Autodesk Inventor part; units mm, degrees
ref_plane "YZ Plane" through (0, 0, 0) normal (1, 0, 0) x (0, 1, 0)
ref_plane "XZ Plane" through (0, 0, 0) normal (0, 1, 0) x (-1, 0, 0)
ref_plane "XY Plane" through (0, 0, 0) normal (0, 0, 1) x (1, 0, 0)
sketch "Sketch1" plane through (0, 0, 0) normal (0, 1, 0) x (-1, 0, 0)
  line L0 (0, 0) -> (-50.8, 0)
  line L1 (-50.8, 0) -> (-50.8, -88.9)
  line L2 (-50.8, -88.9) -> (0, -88.9)
  line L3 (0, -88.9) -> (0, 0)
  dimension "d0" = 50.8
  dimension "d1" = 88.9
extrude "Extrusion1" add sketch "Sketch1" along normal blind 12.7
sketch "Sketch2" plane through (0, 12.7, 0) normal (0, 1, 0) x (1, 0, 0)
  line L0 (50.8, 0) -> (50.8, 88.9)
  line L1 (50.8, 88.9) -> (0, 88.9)
  line L2 (0, 88.9) -> (0, 0)
  line L3 (6.35, 88.9) -> (44.45, 88.9)
  line L4 (44.45, 88.9) -> (44.45, 69.85)
  line L5 (44.45, 69.85) -> (6.35, 69.85)
  line L6 (6.35, 69.85) -> (6.35, 88.9)
  line L7 (6.35, 79.375) -> (0, 79.375) construction
  line L8 (44.45, 79.375) -> (50.8, 79.375) construction
  circle A0 centre (25.4, 69.85) radius 19.05
  dimension "d4" = 19.05
  dimension "d5" = 6.35
extrude "Extrusion2" add sketch "Sketch2" along normal blind 12.7
sketch "Sketch3" plane through (0, 25.4, 0) normal (0, 1, 0) x (1, 0, 0)
  arc A0 (6.35, 69.85) -> (44.45, 69.85) centre (25.4, 69.85) ccw
  circle A1 centre (25.4, 69.85) radius 12.7
  point P0 (0, 0)
  dimension "d8" = 25.4
extrude "Extrusion3" add sketch "Sketch3" along normal blind 12.7
sketch "Sketch6" plane through (0, 12.7, 0) normal (0, 1, 0) x (1, 0, 0)
  line L0 (0, 88.9) -> (0, 0)
  line L1 (0, 0) -> (50.8, 0)
  line L2 (50.8, 0) -> (50.8, 88.9)
  line L3 (44.45, 88.9) -> (44.45, 6.35) construction
  line L4 (44.45, 6.35) -> (6.35, 6.35) construction
  line L5 (6.35, 6.35) -> (6.35, 88.9) construction
  line L6 (6.35, 38.1) -> (44.45, 38.1) construction
  dimension "d35" = 6.35
  dimension "d36" = 31.75
hole "Hole3" at (25.4, 38.1, -69.85) direction (0, -1, 0) diameter 19.05 end through all
hole "Hole4" at (6.35, 12.7, -6.35) at (6.35, 12.7, -38.1) at (44.45, 12.7, -6.35) at (44.45, 12.7, -38.1) direction (0, -1, 0) diameter 5.1054 end through all counterbore diameter 9.525 counterbore depth 4.826
properties part number "Holes"
Verification items for the finished model (mm, model axes). A direction names the side the tool comes from. Coordinates: 2 decimals unless noted, no trailing zeros. Loops run counter-clockwise (first coordinate to the right, second up) from the corner with the lowest first, then second, coordinate; pieces in that order, holes last. Notation, with made-up numbers: (84, -16) - (99, -16) arc R10 cw to (99, -8) - close; hole circle Ø2 at (-20.75, -20.5). An arc over 180 degrees is marked (long way). Return JSON: item names as keys, results as strings.
1. Go/stop test with flat-tipped pins: pin 1 (1 mm diameter, centred on x = 42, z = -69.5, fed in from +Y); pin 2 (6 mm diameter, centred on x = 39, z = -21, fed in from +Y); pin 3 (3 mm diameter, centred on x = 46.5, z = -38, fed in from +Y). Record where each tip stops, or that it passes through.
Established:
{"pin 1": "stops at y = 25.4", "pin 2": "stops at y = 12.7", "pin 3": "stops at y = 7.87"}
2. Tool access check on faces 1 (the flat face through (0, 6, -45)), 2 (the flat face through (44.45, 19, -80)), 3 (the flat face through (8, 7.874, -4)). Record the directions out of +Z, -Z, +X, -X, +Y, -Y that give a thin tool (end or side, any length) a straight path to the whole face; none if there is none.
Established:
{"face 1": "+Z, -Z, -X, +Y, -Y", "face 2": "+Z, -Z, +X, +Y", "face 3": "+Y"}
3. Section check D-D, the plane x = 32. Record the boundary of the cut face in (y, z), then the cut area to 3 significant figures.
Established:
{"outline": "(0, -88.9) - (25.4, -88.9) - (25.4, -80.7) - (38.1, -80.7) - (38.1, -76.72) - (0, -76.72) - close; (0, -62.98) - (38.1, -62.98) - (38.1, -59) - (25.4, -59) - (25.4, -51.98) - (12.7, -51.98) - (12.7, 0) - (0, 0) - close", "area": "1,350 mm2"}
4. Mould release check, pull along Z, two halves, no side actions. Record for faces 4 (the cylindrical face through (41.23, 10.25, -41.61)), 5 (the flat face through (26, 13, -88.9)), 6 (the flat face through (26, 0, -44)): +Z half, -Z half, draft (parallel to the pull), parting line (faces both ways), or undercut.
Established:
{"face 4": "undercut", "face 5": "-Z half", "face 6": "draft"}
5. Section check A-A, the plane x = 25.4. Record the boundary of the cut face in (y, z) (3 decimals).
Established:
{"outline": "(0, -88.9) - (25.4, -88.9) - (25.4, -82.55) - (38.1, -82.55) - (38.1, -79.375) - (0, -79.375) - close; (0, -60.325) - (38.1, -60.325) - (38.1, -57.15) - (25.4, -57.15) - (25.4, -50.8) - (12.7, -50.8) - (12.7, 0) - (0, 0) - close"}
6. Section check B-B, the plane y = 3.5. Record the boundary of the cut face in (x, z) (3 decimals).
Established:
{"outline": "(0, -88.9) - (50.8, -88.9) - (50.8, 0) - (0, 0) - close; hole circle Ø5.105 at (6.35, -38.1); hole circle Ø5.105 at (6.35, -6.35); hole circle Ø19.05 at (25.4, -69.85); hole circle Ø5.105 at (44.45, -38.1); hole circle Ø5.105 at (44.45, -6.35)"}
7. Thickness scan on L1, parallel to X at y = 3, z = -38; L2, parallel to X at y = 8.95, z = -6.35; L3, parallel to Z at x = 44.45, y = 4.5. Record the ranges inside material, lowest first.
Established:
{"L1": "x = 0 to 3.8, 8.9 to 41.9, 47 to 50.8", "L2": "x = 0 to 1.59, 11.11 to 39.69, 49.21 to 50.8", "L3": "z = -88.9 to -40.65, -35.55 to -8.9, -3.8 to 0"}
8. Section check C-C, the plane z = -77. Record the boundary of the cut face in (x, y).
Established:
{"outline": "(0, 0) - (19.11, 0) - (19.11, 38.1) - (14.9, 38.1) - (14.9, 25.4) - (6.35, 25.4) - (6.35, 12.7) - (0, 12.7) - close; (31.69, 0) - (50.8, 0) - (50.8, 12.7) - (44.45, 12.7) - (44.45, 25.4) - (35.9, 25.4) - (35.9, 38.1) - (31.69, 38.1) - close"}
